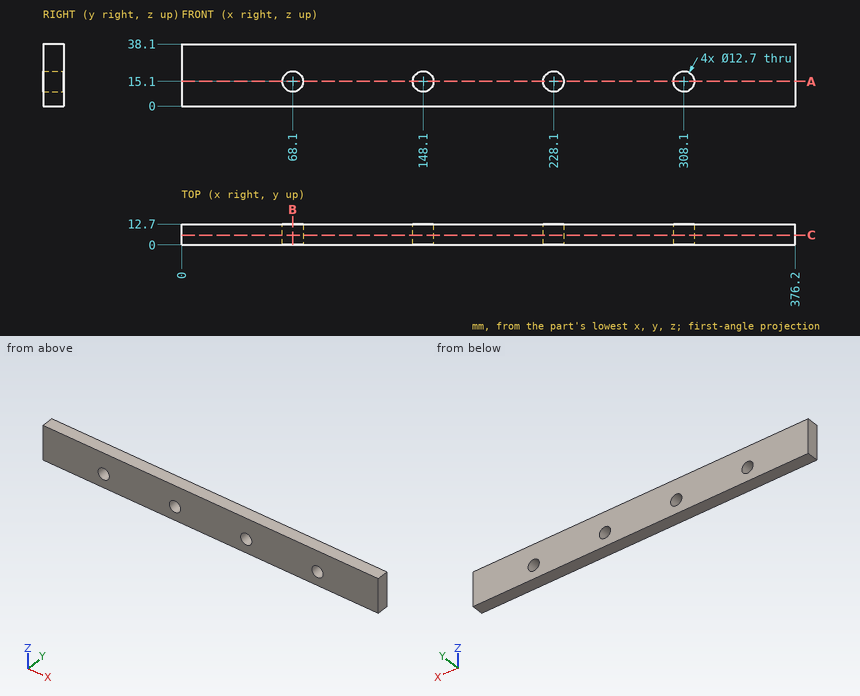
Geometry check sheet. Reference: drawing and pictorial views, mm from the part's lowest x, y, z. Coordinates: 2 decimals unless noted, no trailing zeros. Loops run counter-clockwise (first coordinate to the right, second up) from the corner with the lowest first, then second, coordinate; pieces in that order, holes last. Notation, with made-up numbers: (39, 6.5) - (47, 6.5) arc R14 ccw to (47, 29.5) - close; hole circle Ø2 at (16, 11.5). An arc over 180 degrees is marked (long way). Return JSON: item names as keys, results as strings.
1. Section check C-C, the plane y = 6. Record the boundary of the cut face in (x, z).
Established:
{"outline": "(0, 0) - (376.2, 0) - (376.2, 38.1) - (0, 38.1) - close; hole circle Ø12.7 at (68.1, 15.1); hole circle Ø12.7 at (148.1, 15.1); hole circle Ø12.7 at (228.1, 15.1); hole circle Ø12.7 at (308.1, 15.1)"}
2. Thickness scan on L1, parallel to Z at x = 308.1, y = 5; L2, parallel to X at y = 5.75, z = 14; L3, parallel to X at y = 7, z = 19. Record the ranges inside material, lowest first.
Established:
{"L1": "z = 0 to 8.75, 21.45 to 38.1", "L2": "x = 0 to 61.85, 74.35 to 141.85, 154.35 to 221.85, 234.35 to 301.85, 314.35 to 376.2", "L3": "x = 0 to 63.09, 73.11 to 143.09, 153.11 to 223.09, 233.11 to 303.09, 313.11 to 376.2"}
3. Go/stop test with flat-tipped pins: pin 1 (4 mm diameter, centred on x = 259, z = 23.5, fed in from -Y); pin 2 (7.5 mm diameter, centred on x = 148.1, z = 15.1, fed in from +Y). Record where each tip stops, or that it passes through.
Established:
{"pin 1": "stops at y = 0", "pin 2": "passes through"}
4. Section check B-B, the plane x = 68.1. Record the boundary of the cut face in (y, z).
Established:
{"outline": "(0, 0) - (12.7, 0) - (12.7, 8.75) - (0, 8.75) - close; (0, 21.45) - (12.7, 21.45) - (12.7, 38.1) - (0, 38.1) - close"}
5. Section check A-A, the plane z = 15.1. Record the boundary of the cut face in (x, y), then the cut area to 3 significant figures.
Established:
{"outline": "(0, 0) - (61.75, 0) - (61.75, 12.7) - (0, 12.7) - close; (74.45, 0) - (141.75, 0) - (141.75, 12.7) - (74.45, 12.7) - close; (154.45, 0) - (221.75, 0) - (221.75, 12.7) - (154.45, 12.7) - close; (234.45, 0) - (301.75, 0) - (301.75, 12.7) - (234.45, 12.7) - close; (314.45, 0) - (376.2, 0) - (376.2, 12.7) - (314.45, 12.7) - close", "area": "4,130 mm2"}
